Work out the finished part from the listing and answer in its coordinate system (mm). A direction names the side the tool comes from. Coordinates: 2 decimals unless noted, no trailing zeros. Loops run counter-clockwise (first coordinate to the right, second up) from the corner with the lowest first, then second, coordinate; pieces in that order, holes last. Notation, with made-up numbers: (53, -31.75) - (88, -31.75) arc R24 ccw to (88, -18.75) - close; hole circle Ø4 at (88, 60). An arc over 180 degrees is marked (long way). Write each question's results on one line, items separated by ' | '. Start each with the question number.
Item 1: For a pull along X with two mould halves and no side action, classify faces 1 (the face through (14.5, 0, 8)), 2 (the face through (-9.22, -33.67, 7.4)), 3 (the face through (9.03, -33.73, 7.4)) as +X half, -X half, draft (parallel to the pull), parting line (faces both ways), or undercut.
Item 2: Section D-D, the plane y = -25.4 is taken. Write down the section's boundary in (x, z), plus the area to 3 significant figures.
Item 3: Section B-B, the plane y = -1 is taken. Write down the section's boundary in (x, z).
Item 4: A tool of negligible diameter and unlimited length cuts with its end or side. For faces 4 (the face through (12.696, -13.289, 8.591)), 5 (the face through (0, 17, 7)), from which of +Z, -Z, +X, -X, +Y, -Y can it reach the whole face along a straight path? Write none if from no direction.
Item 5: Section A-A, the plane z = 4 is taken. Write down the section's boundary in (x, y), plus the area to 3 significant figures.
Item 6: Each of these flat-tipped pins is pushed along its axis until it touches: pin 1 Ø1.5 at (y, z) = (4, 5) entering from -X; pin 2 Ø1 at (x, z) = (-19, 10) entering from -Y; pin 3 Ø3 at (x, y) = (2, 11.5) entering from +Z; pin 4 Ø7.5 at (x, y) = (0, -25.4) entering from -Z. Where does it stop, or does it pass through?
Item 7: Section C-C, the plane x = 0 is taken. Write down the section's boundary in (y, z), plus the area to 3 significant figures.
Item 8: Consider probe 1 along Y at (x, z) = (1.5, 11); probe 2 along X at (y, z) = (-2, 12.5); probe 3 along Y at (x, z) = (-2, 7). Determine where each line is inside the solid, lowest interval first. Write a range as [from, to].
from build123d import *

# Parameters (mm, degrees)
SKETCH3_R           = 2.25
SKETCH3_W           = 29
SKETCH3_H           = 30
SKETCH3_R_2         = 9
SKETCH3_R_3         = 6.75
SKETCH3_R_4         = 4.3
BOSS_EXTRUDE1_DEPTH = 15
SKETCH3_3_W         = 29
SKETCH3_3_H         = 30
SKETCH3_3_R         = 7
BOSS_EXTRUDE2_DEPTH = 2
CUT_EXTRUDE1_START  = 13
SKETCH3_4_R         = 6.75
SKETCH3_4_R_2       = 4.3
CUT_EXTRUDE1_DEPTH  = 2
FILLET1_R           = 6
FILLET2_R           = 12


with BuildPart() as part:
    # Sketch3 → Boss-Extrude1 (new body)
    # profile 1 of 3: a face of its own
    with BuildSketch(Plane.XY):
        with BuildLine():
            Line((16.5, 17), (-16.5, 17))
            Line((-16.5, 17), (-24.05, 3.333333333))
            Line((-24.05, 3.333333333), (-24.05, -29.088230031))
            Line((-24.05, -29.088230031), (-2.657112786, -35.698822689))
            ThreePointArc((-2.657112786, -35.698822689), (-5.342564222, -19.857278996), (9, -27.1))
            ThreePointArc((9, -27.1), (7.242721004, -32.442564222), (2.657112786, -35.698822689))
            Line((2.657112786, -35.698822689), (24.05, -29.088230031))
            Line((24.05, -29.088230031), (24.05, 3.333333333))
            Line((24.05, 3.333333333), (16.5, 17))
        make_face()
        with Locations((-19.05, -25.4)):
            Circle(SKETCH3_R, mode=Mode.SUBTRACT)
        with Locations((19.05, -25.4)):
            Circle(SKETCH3_R, mode=Mode.SUBTRACT)
        with Locations((-19.05, 0)):
            Circle(SKETCH3_R, mode=Mode.SUBTRACT)
        Rectangle(SKETCH3_W, SKETCH3_H, mode=Mode.SUBTRACT)
        with Locations((19.05, 0)):
            Circle(SKETCH3_R, mode=Mode.SUBTRACT)
    # profile 2 of 3: a face of its own
    with BuildSketch(Plane.XY):
        with Locations((0, -27.1)):
            Circle(SKETCH3_R_2)
        with Locations((0, -27.1)):
            Circle(SKETCH3_R_3, mode=Mode.SUBTRACT)
    # profile 3 of 3: a face of its own
    with BuildSketch(Plane.XY):
        with Locations((0, -27.1)):
            Circle(SKETCH3_R_3)
        with Locations((0, -25.4)):
            Circle(SKETCH3_R_4, mode=Mode.SUBTRACT)
    extrude(amount=BOSS_EXTRUDE1_DEPTH)

    # Sketch3<3> → Boss-Extrude2 (add)
    with BuildSketch(Plane.XY):
        Rectangle(SKETCH3_3_W, SKETCH3_3_H)
        Circle(SKETCH3_3_R, mode=Mode.SUBTRACT)
    extrude(amount=BOSS_EXTRUDE2_DEPTH)

    # Sketch3<4> → Cut-Extrude1 (cut)
    with BuildSketch(Plane.XY.offset(CUT_EXTRUDE1_START)):
        with Locations((0, -27.1)):
            Circle(SKETCH3_4_R)
        with Locations((0, -25.4)):
            Circle(SKETCH3_4_R_2, mode=Mode.SUBTRACT)
    extrude(amount=CUT_EXTRUDE1_DEPTH, mode=Mode.SUBTRACT)

    # Fillet1
    fillet1_edges = [part.edges().sort_by_distance(p)[0] for p in [
        (-14.5, 15, 8.5),
        (-14.5, -15, 8.5),
        (14.5, -15, 8.5),
        (14.5, 15, 8.5),
    ]]
    fillet(fillet1_edges, radius=FILLET1_R)

    # Fillet2
    fillet2_edges = [part.edges().sort_by_distance(p)[0] for p in [
        (-24.05, -29.088230031, 7.5),
        (-24.05, 3.333333333, 7.5),
        (-16.5, 17, 7.5),
        (16.5, 17, 7.5),
        (24.05, 3.333333333, 7.5),
        (24.05, -29.088230031, 7.5),
    ]]
    fillet(fillet2_edges, radius=FILLET2_R)


solid = part.part
Answer key:
1) face 1: undercut | face 2: -X half | face 3: +X half
2) outline: (-22.88, 0) - (-21.3, 0) - (-21.3, 15) - (-22.88, 15) - close; (-16.8, 0) - (-4.3, 0) - (-4.3, 13) - (-6.53, 13) - (-6.53, 15) - (-16.8, 15) - close; (4.3, 0) - (16.8, 0) - (16.8, 15) - (6.53, 15) - (6.53, 13) - (4.3, 13) - close; (21.3, 0) - (22.88, 0) - (22.88, 15) - (21.3, 15) - close | area: 414 mm^2
3) outline: (-24.05, 0) - (-21.07, 0) - (-21.07, 15) - (-24.05, 15) - close; (-17.03, 0) - (-6.93, 0) - (-6.93, 2) - (-14.5, 2) - (-14.5, 15) - (-17.03, 15) - close; (6.93, 0) - (17.03, 0) - (17.03, 15) - (14.5, 15) - (14.5, 2) - (6.93, 2) - close; (21.07, 0) - (24.05, 0) - (24.05, 15) - (21.07, 15) - close
4) face 4: +Z | face 5: +Z, -Z, +X, -X, +Y
5) outline: (-24.05, -20.24) arc R12 ccw to (-15.59, -31.7) - (-2.66, -35.7) arc R9 ccw to (2.66, -35.7) - (15.59, -31.7) arc R12 ccw to (24.05, -20.24) - (24.05, 0.24) arc R12 ccw to (22.55, 6.04) - (19.92, 10.8) arc R12 ccw to (9.42, 17) - (-9.42, 17) arc R12 ccw to (-19.92, 10.8) - (-22.55, 6.04) arc R12 ccw to (-24.05, 0.24) - close; hole circle Ø4.5 at (-19.05, -25.4); hole circle Ø4.5 at (-19.05, 0); hole (-14.5, -9) arc R6 ccw to (-8.5, -15) - (8.5, -15) arc R6 ccw to (14.5, -9) - (14.5, 9) arc R6 ccw to (8.5, 15) - (-8.5, 15) arc R6 ccw to (-14.5, 9) - close; hole circle Ø8.6 at (0, -25.4); hole circle Ø4.5 at (19.05, -25.4); hole circle Ø4.5 at (19.05, 0) | area: 1,280 mm^2
6) pin 1: stops at x = -23.67 | pin 2: stops at y = -30.36 | pin 3: stops at z = 2 | pin 4: passes through
7) outline: (-36.1, 0) - (-29.7, 0) - (-29.7, 13) - (-33.85, 13) - (-33.85, 15) - (-36.1, 15) - close; (-21.1, 0) - (-7, 0) - (-7, 2) - (-15, 2) - (-15, 15) - (-20.35, 15) - (-20.35, 13) - (-21.1, 13) - close; (7, 0) - (17, 0) - (17, 15) - (15, 15) - (15, 2) - (7, 2) - close | area: 240 mm^2
8) probe 1: y = [-35.97, -29.43], [-21.37, -15], [15, 17] | probe 2: x = [-24.05, -20.08], [-18.02, -14.5], [14.5, 18.02], [20.08, 24.05] | probe 3: y = [-35.87, -29.21], [-21.59, -15], [15, 17]
